Design review of the part built by this model. Coordinates are the model's own, in mm. Face numbers are marked on the shaded views. Coordinates: 2 decimals unless noted, no trailing zeros. Order: outer loops, then holes, each group sorted by start corner. A loop starts at its lowest first (then second) coordinate and runs counter-clockwise, first axis right, second up. Notation, with made-up numbers: (-29.75, 36) -> (-17.75, 36) arc R16 cw to (-17.75, 63) -> close; hole circle Ø1 at (20.5, 29.25). An arc over 180 degrees is marked (long way). Write item = value, one per line.
```python
from build123d import *

# Parameters (mm, degrees)
F0_R     = 7
F1_DEPTH = 54
F3_DEPTH = 57.001


with BuildPart() as f1:
    # F0 (on Front) → F1 (new body)
    with BuildSketch(Plane.XZ):
        Polygon((9.345292, 57), (-52.654708, 57), (-52.654708, 46), (-30.654708, 28.847458), (6.345292, 0), (68.345292, 0), (68.345292, 11), align=None)
        with Locations((24.345292, 12)):
            Circle(F0_R, mode=Mode.SUBTRACT)
        with Locations((-8.654708, 41)):
            Circle(F0_R, mode=Mode.SUBTRACT)
        Polygon((-30.654708, 28.847458), (-52.654708, 46), (-52.654708, 0), (-30.654708, 0), align=None)
        Polygon((68.345292, 57), (9.345292, 57), (68.345292, 11), align=None)
        Polygon((6.345292, 0), (-30.654708, 28.847458), (-30.654708, 0), align=None)
    extrude(amount=F1_DEPTH)

    # F2 (on face) → F3 (cut, through all)
    with BuildSketch(Plane.XY.offset(57)):
        Polygon((68.345292, -22), (-30.654708, -54), (68.345292, -54), align=None)
    extrude(amount=-F3_DEPTH, mode=Mode.SUBTRACT)


solid = f1.part
```
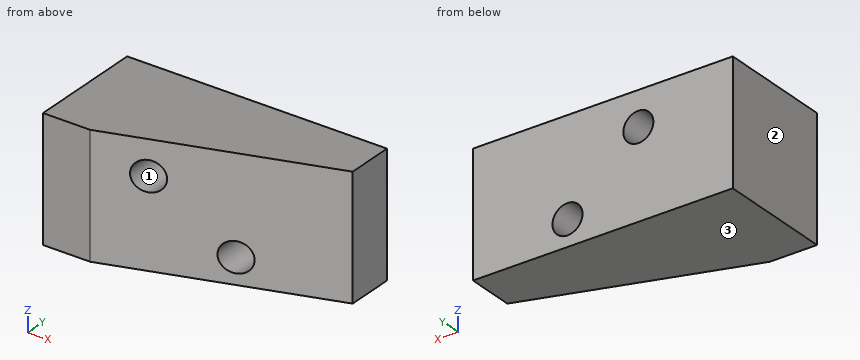
(1) The part is to be moulded in two halves that separate along Z. For the marked faces 1, 2 and 3, say which applies: released by +Z, released by -Z, zero draft, split by the parting line, or undercut.
Report:
face_1 = undercut
face_2 = zero draft
face_3 = released by -Z
(2) We need section A-A (x = 19). Write out the cut boundary in (y, z).
Report:
outline = (-37.95, 0) -> (0, 0) -> (0, 7.48) -> (-37.95, 7.48) -> close; (-37.95, 16.52) -> (0, 16.52) -> (0, 57) -> (-37.95, 57) -> close
(3) Insertion check: pin 1 (12 mm diameter, centred on x = -9, z = 22.5, fed in from -Y); pin 2 (1 mm diameter, centred on x = 33, z = 40.5, fed in from -Y); pin 3 (2 mm diameter, centred on x = -26.5, z = 18, fed in from -Y). Each pin has a flat end and moves straight along its axis. Give the tip position at first contact, or say it passes through.
Report:
pin_1 = -48.94
pin_2 = -33.59
pin_3 = -52.98
(4) We need section C-C (y = -12). Write out the cut boundary in (x, z), and give its area (3 significant figures).
Report:
outline = (-52.65, 0) -> (68.35, 0) -> (68.35, 57) -> (-52.65, 57) -> close; hole circle Ø14 at (-8.65, 41); hole circle Ø14 at (24.35, 12)
area = 6,590 mm²
(5) For L1, parallel to X at y = -8, z = 12; L2, parallel to Z at x = 24.5, y = -18; L3, parallel to Z at x = -7, y = -13.5, list the stretches that pass through material, from the lowest coordinate up.
Report:
L1 = -52.65 to 17.35, 31.35 to 68.35
L2 = 0 to 5, 19 to 57
L3 = 0 to 34.2, 47.8 to 57
(6) We need section D-D (z = 52). Write out the cut boundary in (x, y), and give its area (3 significant figures).
Report:
outline = (-52.65, -54) -> (-30.65, -54) -> (68.35, -22) -> (68.35, 0) -> (-52.65, 0) -> close
area = 4,950 mm²
(7) We need section B-B (z = 41). Write out the cut boundary in (x, y).
Report:
outline = (-52.65, -54) -> (-30.65, -54) -> (-15.65, -49.15) -> (-15.65, 0) -> (-52.65, 0) -> close; (-1.65, -44.63) -> (68.35, -22) -> (68.35, 0) -> (-1.65, 0) -> close
